Verification items for the finished model (mm, model axes). A direction names the side the tool comes from. Coordinates: 2 decimals unless noted, no trailing zeros. Order: outer loops, then holes, each group sorted by start corner. A loop starts at its lowest first (then second) coordinate and runs counter-clockwise, first axis right, second up.
Q1. Draft check along Z on faces 1 (the flat face through (0, -11, 21)), 2 (the cylindrical face through (9.7, -11.3, 24.8)), 3 (the flat face through (6, -8, 0)), 4 (the flat face through (15, -11, 4.57)). Enter one of: pulls with the +Z half, pulls with the -Z half, needs draft (parallel to the pull), parting line crosses it, or undercut.
Q2. Depth check by flat-ended pin: P1, Ø1, axis at y = -8.5, z = 10.5, coming from the +X side; P2, Ø4, axis at y = -7.5, z = 26, coming from the -X side; P3, Ø8, axis at x = 4, y = -10, coming from the +Z side; P4, Ø4, axis at y = -14.88, z = 25.11, coming from the -X side. Enter the tip coordinate at first touch or a pass-through.
Q3. Cross-section at C-C, the plane x = 16.25. Record the boundary of the cut face in (y, z), and give its area (3 significant figures).
Q4. Cross-section at D-D, the plane z = 12. Record the boundary of the cut face in (x, y).
Q5. Cross-section at B-B, the plane x = 5.75. Record the boundary of the cut face in (y, z) (1 decimal), and give its area (3 significant figures).
Q6. Cross-section at A-A, the plane y = -2.25. Record the boundary of the cut face in (x, z).
Q7. Set-up check for faces 5 (the flat face through (15.581, -5.054, 2.253)), 6 (the cylindrical face through (6.085, -9.604, 35.46)): record each of +Z, -Z, +X, -X, +Y, -Y from which the full face is reachable in a straight line by a thin tool's end or side.
Q8. Thickness scan on line 1 (X direction, y = -1, z = 13); line 2 (Z direction, x = -4.25, y = -6); line 3 (X direction, y = -10.5, z = 23). Record the ranges inside material, lowest first.
from build123d import *

# Parameters (mm, degrees)
F1_DEPTH     = 5
F3_DEPTH     = 2.2
F5_DEPTH     = 5
F6_R         = 14.1038356314
F7_W         = 8.643694222
F7_H         = 4.569907207
F8_DEPTH     = 6.858
F10_DEPTH    = 25.654
F9_R         = 1.5875
F11_DEPTH    = 26.924
F12_R        = 1.5875
F13_DEPTH    = 9.5758
F14_T4_DEPTH = 4.569907207
F14_T9_DEPTH = 4.569907207
F15_R        = 1.5875
F16_DEPTH    = 18.034


# Not quite as in the source:
# - a fillet or chamfer that OpenCascade refuses, or shapes differently, is made with other operations: its cross-section is extruded or revolved along the edge and cut away or added


with BuildPart() as f1:
    # F0 (on Right) → F1 (new body)
    with BuildSketch(Plane.YZ):
        with BuildLine():
            Line((-17.1746751294, 0), (0, 0))
            Line((0, 0), (0, 15))
            ThreePointArc((0, 15), (-10, 25), (0, 35))
            Line((0, 35), (0, 42.1679355204))
            Line((0, 42.1679355204), (-17.1746751294, 42.1679355204))
            Line((-17.1746751294, 42.1679355204), (-17.1746751294, 0))
        make_face()
    extrude(amount=F1_DEPTH)

    # F2 (on face) → F3 (join)
    with BuildSketch(Plane.YZ.offset(5)):
        with BuildLine():
            ThreePointArc((0, 10.8), (-14.2, 25), (0, 39.2))
            Line((0, 39.2), (0, 42.1679355204))
            Line((0, 42.1679355204), (-17.1746751294, 42.1679355204))
            Line((-17.1746751294, 42.1679355204), (-17.1746751294, 0))
            Line((-17.1746751294, 0), (0, 0))
            Line((0, 0), (0, 10.8))
        make_face()
    extrude(amount=F3_DEPTH)

    # F4 (on face) → F5 (join)
    with BuildSketch(Plane.YZ.offset(7.2)):
        with BuildLine():
            ThreePointArc((0, 10.8), (-14.2, 25), (0, 39.2))
            Line((0, 39.2), (0, 42.1679355204))
            Line((0, 42.1679355204), (-17.1746751294, 42.1679355204))
            Line((-17.1746751294, 42.1679355204), (-17.1746751294, 0))
            Line((-17.1746751294, 0), (0, 0))
            Line((0, 0), (0, 10.8))
        make_face()
        with BuildLine():
            ThreePointArc((0, 13.7), (-11.3, 25), (0, 36.3))
            Line((0, 36.3), (0, 39.2))
            ThreePointArc((0, 39.2), (-14.2, 25), (0, 10.8))
            Line((0, 10.8), (0, 13.7))
        make_face()
    extrude(amount=F5_DEPTH)

    # F6
    f6_edges = [f1.edges().sort_by_distance(p)[0] for p in [
        (6.1, -17.174675, 42.167936),
    ]]
    fillet(f6_edges, radius=F6_R)

    # F7 (on face) → F8 (join)
    with BuildSketch(Plane.YZ.offset(12.2)):
        with Locations((-12.8528280184, 2.2849536035)):
            Rectangle(F7_W, F7_H)
    extrude(amount=F8_DEPTH)

    # F10 (add): a face of the model
    f10_faces = [f1.faces().sort_by_distance(p)[0] for p in [
        (19.058, -12.8528280184, 2.2849536035),
    ]]
    extrude(f10_faces, amount=-F10_DEPTH)

    # F9 (on face) → F11 (cut)
    with BuildSketch(Plane.XY.offset(4.569907207)):
        with Locations((15.894247219, -12.8528280184)):
            Circle(F9_R)
    extrude(amount=-F11_DEPTH, mode=Mode.SUBTRACT)

    # F12 (on face) → F13 (cut)
    with BuildSketch(Plane.XY.offset(4.569907207)):
        with Locations((-3.329155501, -12.8116961569)):
            Circle(F12_R)
    extrude(amount=-F13_DEPTH, mode=Mode.SUBTRACT)

    # F14: chamfer of 6.858 on 2 edges, made by hand


with BuildPart() as f14_tool2:
    # F14_s3 → F14_t4 (new body)
    with BuildSketch(Plane.XY):
        Polygon((12.2, -1.6729809074), (19.058, -8.5309809074), (12.2, -8.5309809074), align=None)
    extrude(amount=F14_T4_DEPTH)

    split(bisect_by=Plane.YZ.offset(19.058), keep=Keep.BOTTOM)


with BuildPart() as f1_1:
    add(f1.part)

    # F14_t1: union F14_tool2
    add(f14_tool2.part)


with BuildPart() as f14_tool7:
    # F14_s8 → F14_t9 (new body)
    with BuildSketch(Plane.XY):
        Polygon((0, -1.6729809074), (-6.858, -8.5309809074), (0, -8.5309809074), align=None)
    extrude(amount=F14_T9_DEPTH)

    split(bisect_by=Plane.YZ.offset(-6.596), keep=Keep.TOP)


with BuildPart() as f1_2:
    add(f1_1.part)

    # F14_t6: union F14_tool7
    add(f14_tool7.part)

    # F15 (on face) → F16 (cut)
    with BuildSketch(Plane.YZ.offset(12.2)):
        with Locations((-14.881552197, 25.1055490226)):
            Circle(F15_R)
    extrude(amount=-F16_DEPTH, mode=Mode.SUBTRACT)


solid = f1_2.part
Check values:
1. face 1: needs draft
1. face 2: undercut
1. face 3: pulls with the -Z half
1. face 4: pulls with the +Z half
2. P1: stops at x = 12.2
2. P2: passes through
2. P3: stops at z = 41.86
2. P4: stops at x = 0
3. outline: (-17.17, 0) - (-14.4, 0) - (-14.4, 4.57) - (-17.17, 4.57) - close; (-11.31, 0) - (-5.72, 0) - (-5.72, 4.57) - (-11.31, 4.57) - close
3. area: 38.2 mm2
4. outline: (0, -17.17) - (12.2, -17.17) - (12.2, 0) - (7.2, 0) - (7.2, -5.71) - (5, -5.71) - (5, 0) - (0, 0) - close
5. outline: (-17.2, 0) - (0, 0) - (0, 10.8) arc R14.2 cw to (-14.1, 23.7) arc R1.6 cw (long way) to (-14.1, 26.5) arc R14.2 cw to (0, 39.2) - (0, 42.2) - (-3.1, 42.2) arc R14.1 ccw to (-17.2, 28.1) - close
5. area: 359 mm2
6. outline: (-0.58, 0) - (12.78, 0) - (12.78, 4.57) - (12.2, 4.57) - (12.2, 13.93) - (7.2, 13.93) - (7.2, 10.98) - (5, 10.98) - (5, 15.26) - (0, 15.26) - (0, 4.57) - (-0.58, 4.57) - close; (0, 34.74) - (5, 34.74) - (5, 39.02) - (7.2, 39.02) - (7.2, 36.07) - (12.2, 36.07) - (12.2, 42.17) - (0, 42.17) - close
7. face 5: +Z, -Z, +X, +Y
7. face 6: +Y
8. line 1: x = 0 to 5, 7.2 to 12.2
8. line 2: z = 0 to 4.57
8. line 3: x = 0 to 5
